```python
from build123d import *

# Parameters (mm, degrees)
AUFSATZ_LINEAR_AUSTRAGEN1_DEPTH      = 10.25
AUFSATZ_LINEAR_AUSTRAGEN1_DEPTH_BACK = 10.25
SKIZZE2_R                            = 4
AUFSATZ_LINEAR_AUSTRAGEN2_DEPTH      = 20


with BuildPart() as part:
    # Skizze1 → Aufsatz-Linear austragen1 (new body, two sides)
    with BuildSketch(Plane(origin=(0, 0, 0), x_dir=(1, 0, 0), z_dir=(0, 1, 0))) as aufsatz_linear_austragen1_sk:
        Polygon((0, 21.25), (0, -21.25), (-55.174682453, -21.25), (-66, -15), (-74, -15), (-74, 15), (-66, 15), (-55.174682453, 21.25), align=None)
    extrude(amount=AUFSATZ_LINEAR_AUSTRAGEN1_DEPTH)
    extrude(aufsatz_linear_austragen1_sk.sketch, amount=-AUFSATZ_LINEAR_AUSTRAGEN1_DEPTH_BACK)

    # Skizze2 → Aufsatz-Linear austragen2 (add)
    with BuildSketch(Plane(origin=(0, 0, 0), x_dir=(0, 0, -1), z_dir=(1, 0, 0))):
        Circle(SKIZZE2_R)
    extrude(amount=AUFSATZ_LINEAR_AUSTRAGEN2_DEPTH)


solid = part.part
```
Design review of the part built by this model. Coordinates are the model's own, in mm. A direction names the side the tool comes from. Coordinates: 2 decimals unless noted, no trailing zeros. Loops run counter-clockwise (first coordinate to the right, second up) from the corner with the lowest first, then second, coordinate; pieces in that order, holes last. Notation, with made-up numbers: (-26.75, 81) -> (25.25, 81) arc R28 ccw to (25.25, 111) -> close; hole circle Ø2 at (-6, 38). An arc over 180 degrees is marked (long way). Answer as a JSON object with one key per item and string values.
Q1. Take a section at C-C on x = 6. Give the boundary of the cut face in (y, z), plus the area to 3 significant figures.
Answer block:
{"outline": "circle Ø8 at (0, 0)", "area": "50.3 mm^2"}
Q2. To check wall thickness, follow L1, parallel to X at y = 1.75, z = -13; L2, parallel to Z at x = -67.5, y = -4.25; L3, parallel to X at y = 1, z = -18.5. State the ranges of each line that lie inside material, in increasing order.
Answer block:
{"L1": "x = -74 to 0", "L2": "z = -15 to 15", "L3": "x = -59.94 to 0"}
Q3. Take a section at B-B on z = 0. Give the boundary of the cut face in (x, y), plus the area to 3 significant figures.
Answer block:
{"outline": "(-74, -10.25) -> (0, -10.25) -> (0, -4) -> (20, -4) -> (20, 4) -> (0, 4) -> (0, 10.25) -> (-74, 10.25) -> close", "area": "1,680 mm^2"}
Q4. Take a section at D-D on y = 0. Give the boundary of the cut face in (x, z), plus the area to 3 significant figures.
Answer block:
{"outline": "(-74, -15) -> (-66, -15) -> (-55.17, -21.25) -> (0, -21.25) -> (0, -4) -> (20, -4) -> (20, 4) -> (0, 4) -> (0, 21.25) -> (-55.17, 21.25) -> (-66, 15) -> (-74, 15) -> close", "area": "3,140 mm^2"}
Q5. Tool access review of faces 1 (the cylindrical face through (9.86, -3.905, 0.867)), 2 (the flat face through (-70, 0, -15)), 3 (the flat face through (-70, 0, 15)): name each direction out of +Z, -Z, +X, -X, +Y, -Y from which nothing blocks a thin tool from reaching the whole face with its end or side.
Answer block:
{"face 1": "+X", "face 2": "-Z, -X, +Y, -Y", "face 3": "+Z, -X, +Y, -Y"}
Q6. Clearance check with flat-ended pins moving along their axes: pin 1 Ø8 at (y, z) = (0.5, -9) entering from +X; pin 2 Ø4 at (x, y) = (-69, 2) entering from -Z; pin 3 Ø2.5 at (x, y) = (-71, -3.5) entering from +Z. State where each tip first meets the part, or that it passes through.
Answer block:
{"pin 1": "stops at x = 0", "pin 2": "stops at z = -15", "pin 3": "stops at z = 15"}
Q7. Take a section at A-A on y = 5.25. Give the boundary of the cut face in (x, z), plus the area to 3 significant figures.
Answer block:
{"outline": "(-74, -15) -> (-66, -15) -> (-55.17, -21.25) -> (0, -21.25) -> (0, 21.25) -> (-55.17, 21.25) -> (-66, 15) -> (-74, 15) -> close", "area": "2,980 mm^2"}
